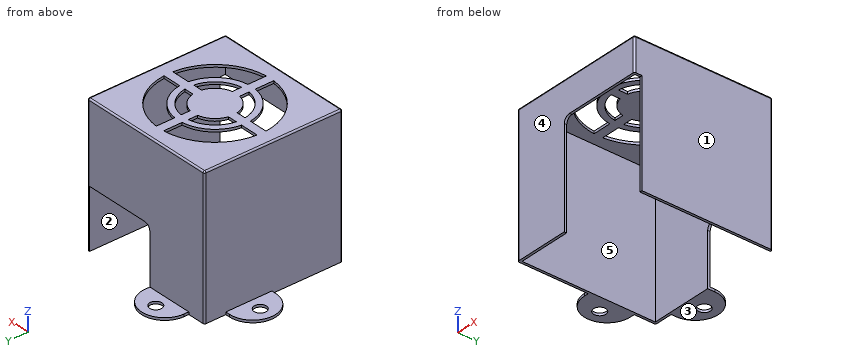
```python
from build123d import *

# Parameters (mm, degrees)
SKETCH1_W           = 45
SKETCH1_H           = 45
BOSS_EXTRUDE1_DEPTH = 45
SHELL1_T            = -0.8
CUT_EXTRUDE1_DEPTH  = 45
SKETCH3_W           = 34
SKETCH3_H           = 2.5
CUT_EXTRUDE2_DEPTH  = 27
FILLET1_R           = 2
FILLET2_R           = 0.5
FILLET3_R           = 0.5
SKETCH4_R           = 2
BOSS_EXTRUDE2_DEPTH = 0.8
CUT_EXTRUDE4_DEPTH  = 0.8


with BuildPart() as part:
    # Sketch1 → Boss-Extrude1 (new body)
    with BuildSketch(Plane(origin=(0, 0, 0), x_dir=(1, 0, 0), z_dir=(0, 1, 0))):
        with Locations((22.5, -22.5)):
            Rectangle(SKETCH1_W, SKETCH1_H)
    extrude(amount=BOSS_EXTRUDE1_DEPTH)

    # Shell1
    shell1_openings = [part.faces().sort_by_distance(p)[0] for p in [
        (22.5, 22.5, 0),
    ]]
    offset(amount=SHELL1_T, openings=shell1_openings, kind=Kind.INTERSECTION)

    # Sketch2 → Cut-Extrude1 (cut)
    with BuildSketch(Plane.XY.offset(45)):
        with BuildLine():
            Line((21.076744556, 34.415298735), (21.076744556, 40.443643553))
            ThreePointArc((21.076744556, 40.443643553), (9.772077939, 35.227922061), (4.556356447, 23.923255444))
            Line((4.556356447, 23.923255444), (10.584701265, 23.923255444))
            ThreePointArc((10.584701265, 23.923255444), (14.014718626, 30.985281374), (21.076744556, 34.415298735))
        make_face()
        with BuildLine():
            ThreePointArc((40.443643553, 23.923255444), (35.227922061, 35.227922061), (23.923255444, 40.443643553))
            Line((23.923255444, 40.443643553), (23.923255444, 34.415298735))
            ThreePointArc((23.923255444, 34.415298735), (30.985281374, 30.985281374), (34.415298735, 23.923255444))
            Line((34.415298735, 23.923255444), (40.443643553, 23.923255444))
        make_face()
        with BuildLine():
            ThreePointArc((23.923255444, 4.556356447), (35.227922061, 9.772077939), (40.443643553, 21.076744556))
            Line((40.443643553, 21.076744556), (34.415298735, 21.076744556))
            ThreePointArc((34.415298735, 21.076744556), (30.985281374, 14.014718626), (23.923255444, 10.584701265))
            Line((23.923255444, 10.584701265), (23.923255444, 4.556356447))
        make_face()
        with BuildLine():
            Line((10.584701265, 21.076744556), (4.556356447, 21.076744556))
            ThreePointArc((4.556356447, 21.076744556), (9.772077939, 9.772077939), (21.076744556, 4.556356447))
            Line((21.076744556, 4.556356447), (21.076744556, 10.584701265))
            ThreePointArc((21.076744556, 10.584701265), (14.014718626, 14.014718626), (10.584701265, 21.076744556))
        make_face()
        with BuildLine():
            ThreePointArc((23.923255444, 12.601800975), (29.571067812, 15.428932188), (32.398199025, 21.076744556))
            Line((32.398199025, 21.076744556), (29.353783184, 21.076744556))
            ThreePointArc((29.353783184, 21.076744556), (27.449747468, 17.550252532), (23.923255444, 15.646216816))
            Line((23.923255444, 15.646216816), (23.923255444, 12.601800975))
        make_face()
        with BuildLine():
            ThreePointArc((32.398199025, 23.923255444), (29.571067812, 29.571067812), (23.923255444, 32.398199025))
            Line((23.923255444, 32.398199025), (23.923255444, 29.353783184))
            ThreePointArc((23.923255444, 29.353783184), (27.449747468, 27.449747468), (29.353783184, 23.923255444))
            Line((29.353783184, 23.923255444), (32.398199025, 23.923255444))
        make_face()
        with BuildLine():
            Line((21.076744556, 29.353783184), (21.076744556, 32.398199025))
            ThreePointArc((21.076744556, 32.398199025), (15.428932188, 29.571067812), (12.601800975, 23.923255444))
            Line((12.601800975, 23.923255444), (15.646216816, 23.923255444))
            ThreePointArc((15.646216816, 23.923255444), (17.550252532, 27.449747468), (21.076744556, 29.353783184))
        make_face()
        with BuildLine():
            Line((15.646216816, 21.076744556), (12.601800975, 21.076744556))
            ThreePointArc((12.601800975, 21.076744556), (15.428932188, 15.428932188), (21.076744556, 12.601800975))
            Line((21.076744556, 12.601800975), (21.076744556, 15.646216816))
            ThreePointArc((21.076744556, 15.646216816), (17.550252532, 17.550252532), (15.646216816, 21.076744556))
        make_face()
    extrude(amount=-CUT_EXTRUDE1_DEPTH, mode=Mode.SUBTRACT)

    # Sketch3 → Cut-Extrude2 (cut)
    with BuildSketch(Plane(origin=(45, 0, 0), x_dir=(0, 0, -1), z_dir=(1, 0, 0))):
        with Locations((-17, 1.25)):
            Rectangle(SKETCH3_W, SKETCH3_H)
    extrude(amount=-CUT_EXTRUDE2_DEPTH, mode=Mode.SUBTRACT)

    # Fillet1
    fillet1_edges = [part.edges().sort_by_distance(p)[0] for p in [
        (18, 0.4, 34),
    ]]
    fillet(fillet1_edges, radius=FILLET1_R)

    # Fillet2
    fillet2_edges = [part.edges().sort_by_distance(p)[0] for p in [
        (45, 22.5, 45),
        (0, 22.5, 45),
    ]]
    fillet(fillet2_edges, radius=FILLET2_R)

    # Fillet3
    fillet3_edges = [part.edges().sort_by_distance(p)[0] for p in [
        (22.5, 0, 45),
        (22.5, 45, 45),
        (45, 0, 39.25),
        (44.853553391, 0, 44.853553391),
        (0.146446609, 0, 44.853553391),
        (45, 45, 22.25),
        (44.853553391, 45, 44.853553391),
        (0.146446609, 45, 44.853553391),
        (0, 45, 22.25),
        (0, 0, 22.25),
    ]]
    fillet(fillet3_edges, radius=FILLET3_R)

    # Sketch4 → Boss-Extrude2 (add)
    # profile 1 of 2: a face of its own
    with BuildSketch(Plane(origin=(0, 0, 0), x_dir=(-1, 0, 0), z_dir=(0, 0, -1))):
        with BuildLine():
            Line((-21, 45), (-6, 45))
            Line((-6, 45), (-6, 46.5))
            ThreePointArc((-6, 46.5), (-13.5, 54), (-21, 46.5))
            Line((-21, 46.5), (-21, 45))
        make_face()
        with Locations((-13.5, 49.4)):
            Circle(SKETCH4_R, mode=Mode.SUBTRACT)
    # profile 2 of 2: a face of its own
    with BuildSketch(Plane(origin=(0, 0, 0), x_dir=(-1, 0, 0), z_dir=(0, 0, -1))):
        with BuildLine():
            Line((1.5, 38), (0, 38))
            Line((0, 38), (0, 23))
            Line((0, 23), (1.5, 23))
            ThreePointArc((1.5, 23), (9, 30.5), (1.5, 38))
        make_face()
        with Locations((4.4, 30.5)):
            Circle(SKETCH4_R, mode=Mode.SUBTRACT)
    extrude(amount=-BOSS_EXTRUDE2_DEPTH)

    # Sketch5 → Cut-Extrude4 (cut)
    with BuildSketch(Plane(origin=(0, 45, 0), x_dir=(1, 0, 0), z_dir=(0, 1, 0))):
        with BuildLine():
            Line((21, 0), (21, -17.2))
            ThreePointArc((21, -17.2), (21.585786438, -18.614213562), (23, -19.2))
            Line((23, -19.2), (44.2, -19.2))
            Line((44.2, -19.2), (44.2, 0))
            Line((44.2, 0), (21, 0))
        make_face()
    extrude(amount=-CUT_EXTRUDE4_DEPTH, mode=Mode.SUBTRACT)


solid = part.part
```
Can you work these out from the model? Positions are in its coordinate system, mm. Face numbers are marked on the shaded views. A direction names the side the tool comes from. Coordinates: 2 decimals unless noted, no trailing zeros. Loops run counter-clockwise (first coordinate to the right, second up) from the corner with the lowest first, then second, coordinate; pieces in that order, holes last.
Item 1: Suppose I cut it at C-C (y = 7). Please give me the cut outline in (x, z).
Answers below:
outline: (0, 0) - (0.8, 0) - (0.8, 44.2) - (13.35, 44.2) - (13.35, 45) - (0.5, 45) arc R0.5 ccw to (0, 44.5) - close; (21.08, 44.2) - (23.92, 44.2) - (23.92, 45) - (21.08, 45) - close; (31.65, 44.2) - (44.2, 44.2) - (44.2, 0) - (45, 0) - (45, 44.5) arc R0.5 ccw to (44.5, 45) - (31.65, 45) - close
Item 2: Suppose I cut it at B-B (x = 7). Please give me the cut outline in (y, z).
Answers below:
outline: (0, 0) - (0.8, 0) - (0.8, 44.2) - (13.35, 44.2) - (13.35, 45) - (0.5, 45) arc R0.5 ccw to (0, 44.5) - close; (21.08, 44.2) - (23.92, 44.2) - (23.92, 45) - (21.08, 45) - close; (31.65, 44.2) - (44.2, 44.2) - (44.2, 0) - (50.24, 0) - (50.24, 0.8) - (45, 0.8) - (45, 44.5) arc R0.5 ccw to (44.5, 45) - (31.65, 45) - close
Item 3: I'm going to push flat-ended pins straight in: pin 1 (0.6 mm diameter, centred on y = 7.5, z = 45, fed in from +X); pin 2 (2.5 mm diameter, centred on x = 13.5, y = 49.4, fed in from -Z); pin 3 (12 mm diameter, centred on x = 32, y = 24.5, fed in from -Z); pin 4 (10 mm diameter, centred on x = 26.5, z = 24.5, fed in from -Y). Where does each tip first touch, or does it pass through?
Answers below:
pin 1: stops at x = 44.96
pin 2: passes through
pin 3: stops at z = 44.2
pin 4: stops at y = 44.2
Item 4: Which directions (+Z, -Z, +X, -X, +Y, -Y) give clear straight access to the entire face, cutting with the end or side of a thin tool? Please do the marked faces 1 and 2.
Answers below:
face 1: +Z, -Z, +X, +Y, -Y
face 2: -Z
Item 5: Suppose I cut it at A-A (z = 3). Please give me the cut outline in (x, y), then the cut area to 3 significant figures.
Answers below:
outline: (0, 0.5) arc R0.5 ccw to (0.5, 0) - (18, 0) - (18, 0.8) - (0.8, 0.8) - (0.8, 44.2) - (21, 44.2) - (21, 45) - (0.5, 45) arc R0.5 ccw to (0, 44.5) - close; (44.2, 2.5) - (45, 2.5) - (45, 44.5) arc R0.5 ccw to (44.5, 45) - (44.2, 45) - close
area: 99.8 mm2
Item 6: Suppose I cut it at D-D (y = 30.5). State how many separate pieces and enclosed holes the cut face has, then the cut area to 3 significant figures.
Answers below:
separate pieces: 6
enclosed holes: 0
area: 91.8 mm2
Item 7: If we mould it in two halves opening along Y, with no side actions, what happens to the marked faces 3, 4 and 5? For each: released by +Y, released by -Y, zero draft, split by the parting line, or undercut.
Answers below:
face 3: zero draft
face 4: released by -Y
face 5: undercut
Item 8: Please list where these lines run through material, in increasing order: L1, parallel to Y at x = 13.5, z = 0.2; L2, parallel to X at y = 3, z = 18.5.
Answers below:
L1: y = 0 to 0.8, 44.2 to 47.4, 51.4 to 54
L2: x = 0 to 0.8, 44.2 to 45
